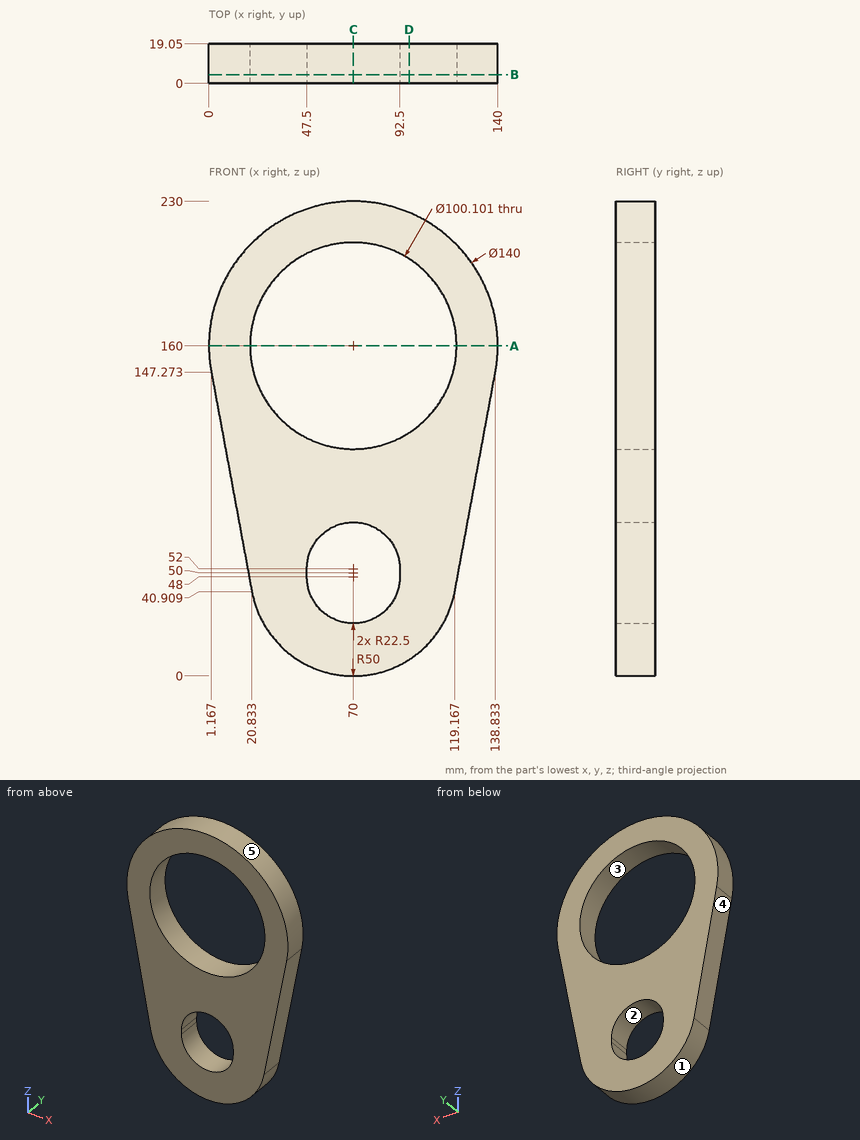
Check sheet for the drawn part. Datum: minimum x, y, z corner. Units: mm. A direction names the side the tool comes from. Give positions to 0.01 mm unless a question says otherwise; leave off trailing zeros. Order: outer loops, then holes, each group sorted by start corner. A loop starts at its lowest first (then second) coordinate and runs counter-clockwise, first axis right, second up. Notation, with made-up numbers: (69.25, 74) -> (122.25, 74) arc R16 ccw to (122.25, 91) -> close; hole circle Ø2 at (76, 68.5). An arc over 180 degrees is marked (long way). Return JSON: item names as keys, results as strings.
1. Material ranges on probe 1 along Z at (x, y) = (70, 9); probe 2 along Z at (x, y) = (66, 10.5) (1 decimal); probe 3 along X at (y, z) = (16.5, 158), recorded low to high. Write a range as [from, to].
From the geometry:
{"probe 1": "[0, 25.5], [74.5, 109.95], [210.05, 230]", "probe 2": "[0.2, 25.9], [74.1, 110.1], [209.9, 229.9]", "probe 3": "[0.03, 19.99], [120.01, 139.97]"}
2. Cross-section at B-B, the plane y = 4.25. Record the cut outline in (x, z), plus the area to 3 significant figures.
From the geometry:
{"outline": "(1.17, 147.27) -> (20.83, 40.91) arc R50 ccw to (119.17, 40.91) -> (138.83, 147.27) arc R70 ccw (long way) to start; hole circle Ø100.1 at (70, 160); hole (47.5, 48) arc R22.5 ccw to (92.5, 48) -> (92.5, 52) arc R22.5 ccw to (47.5, 52) -> close", "area": "15,400 mm^2"}
3. Mould release check, pull along X, two halves, no side actions. Record for the marked faces 3, 4 and 5: +X half, -X half, draft (parallel to the pull), parting line (faces both ways), or undercut.
From the geometry:
{"face 3": "undercut", "face 4": "-X half", "face 5": "parting line"}
4. Cross-section at A-A, the plane z = 160. Record the cut outline in (x, y), plus the area to 3 significant figures.
From the geometry:
{"outline": "(0, 0) -> (19.95, 0) -> (19.95, 19.05) -> (0, 19.05) -> close; (120.05, 0) -> (140, 0) -> (140, 19.05) -> (120.05, 19.05) -> close", "area": "760 mm^2"}
5. Cross-section at C-C, the plane x = 70. Record the cut outline in (y, z).
From the geometry:
{"outline": "(0, 0) -> (19.05, 0) -> (19.05, 25.5) -> (0, 25.5) -> close; (0, 74.5) -> (19.05, 74.5) -> (19.05, 109.95) -> (0, 109.95) -> close; (0, 210.05) -> (19.05, 210.05) -> (19.05, 230) -> (0, 230) -> close"}
6. Cross-section at D-D, the plane x = 97. Record the cut outline in (y, z).
From the geometry:
{"outline": "(0, 7.92) -> (19.05, 7.92) -> (19.05, 117.86) -> (0, 117.86) -> close; (0, 202.14) -> (19.05, 202.14) -> (19.05, 224.58) -> (0, 224.58) -> close"}
7. Go/stop test with flat-tipped pins: P1, Ø10, axis at y = 11, z = 47.5, coming from the +X side; P2, Ø5, axis at x = 24.5, y = 10, coming from the +Z side (1 decimal); P3, Ø3, axis at y = 8, z = 51, coming from the -X side. Record where each tip stops, or that it passes through.
From the geometry:
{"P1": "x = 121.31", "P2": "z = 215.2", "P3": "x = 18.69"}
8. Set-up check for the marked faces 1 and 2: record each of +Z, -Z, +X, -X, +Y, -Y from which the full face is reachable in a straight line by a thin tool's end or side.
From the geometry:
{"face 1": "-Z, +Y, -Y", "face 2": "+Y, -Y"}
